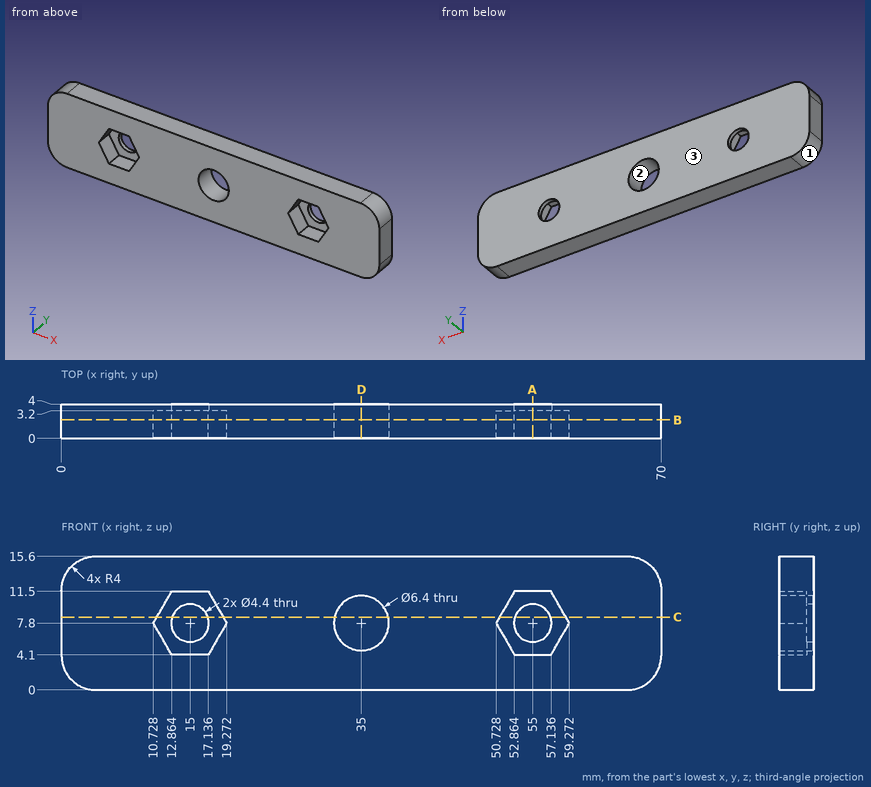
Here's the drawing with two shaded views (mm, measured from the low corner). I have some questions. Round coordinates to 2 decimals unless told otherwise and drop trailing zeros. Loops run counter-clockwise (first coordinate to the right, second up) from the corner with the lowest first, then second, coordinate; pieces in that order, holes last. Notation, with made-up numbers: (-27, 59.25) -> (28, 59.25) arc R11 ccw to (28, 71.25) -> close; hole circle Ø2 at (-6, 28.5). An arc over 180 degrees is marked (long way). Answer as CSV lines item,"result". Start each with the question number.
1. If we mould it in two halves opening along Z, with no side actions, what happens to the marked faces 1, 2 and 3? For each: pulls with the +Z half, pulls with the -Z half, needs draft (parallel to the pull), parting line crosses it, or undercut.
2. Imagine slicing it at C-C on z = 8.5. Write out the boundary of the cut face in (x, y) (1 decimal).
3. I'm going to push a flat-ended pin straight in: P1, Ø3, axis at x = 14, z = 6, coming from the -Y side. Where does the tip first touch, or does it pass through?
4. Imagine slicing it at B-B on y = 2.15. Write out the boundary of the cut face in (x, z), plus the area to 3 significant figures.
5. Imagine slicing it at A-A on x = 55. Write out the boundary of the cut face in (y, z).
6. Imagine slicing it at D-D on x = 35. Write out the boundary of the cut face in (y, z).
7. I need wall thicknesses on probe 1 along X at (y, z) = (3.25, 7.8); probe 2 along Z at (x, y) = (54.5, 0.35); probe 3 along X at (y, z) = (0.65, 10.5) (1 decimal). Which ranges of each line are inside material? Lowest first, please. Write a range as from..to.
Solution:
1,face 1,"pulls with the -Z half"
1,face 2,"undercut"
1,face 3,"needs draft"
2,outline,"(0, 0) -> (11.1, 0) -> (11.1, 3.2) -> (12.9, 3.2) -> (12.9, 4) -> (0, 4) -> close; (17.1, 3.2) -> (18.9, 3.2) -> (18.9, 0) -> (31.9, 0) -> (31.9, 4) -> (17.1, 4) -> close; (38.1, 0) -> (51.1, 0) -> (51.1, 3.2) -> (52.9, 3.2) -> (52.9, 4) -> (38.1, 4) -> close; (57.1, 3.2) -> (58.9, 3.2) -> (58.9, 0) -> (70, 0) -> (70, 4) -> (57.1, 4) -> close"
3,P1,"y = 3.2"
4,outline,"(0, 4) arc R4 ccw to (4, 0) -> (66, 0) arc R4 ccw to (70, 4) -> (70, 11.6) arc R4 ccw to (66, 15.6) -> (4, 15.6) arc R4 ccw to (0, 11.6) -> close; hole (10.73, 7.8) -> (12.86, 4.1) -> (17.14, 4.1) -> (19.27, 7.8) -> (17.14, 11.5) -> (12.86, 11.5) -> close; hole circle Ø6.4 at (35, 7.8); hole (50.73, 7.8) -> (52.86, 4.1) -> (57.14, 4.1) -> (59.27, 7.8) -> (57.14, 11.5) -> (52.86, 11.5) -> close"
4,area,"951 mm²"
5,outline,"(0, 0) -> (4, 0) -> (4, 5.6) -> (3.2, 5.6) -> (3.2, 4.1) -> (0, 4.1) -> close; (0, 11.5) -> (3.2, 11.5) -> (3.2, 10) -> (4, 10) -> (4, 15.6) -> (0, 15.6) -> close"
6,outline,"(0, 0) -> (4, 0) -> (4, 4.6) -> (0, 4.6) -> close; (0, 11) -> (4, 11) -> (4, 15.6) -> (0, 15.6) -> close"
7,probe 1,"0..12.8, 17.2..31.8, 38.2..52.8, 57.2..70"
7,probe 2,"0..4.1, 11.5..15.6"
7,probe 3,"0..12.3, 17.7..33.3, 36.7..52.3, 57.7..70"
